from build123d import *

# Parameters (mm, degrees)
F0_W           = 220
F0_H           = 100
F0_R           = 0.625
F0_W_2         = 50
F0_H_2         = 80
F0_R_2         = 0.6265
F1_DEPTH       = 6.6
F2_SIZE2       = 2
F2_SIZE        = 2
F3_D           = 6.8
F4_D           = 6.6
F4_CBORE_D     = 11.25
F4_CBORE_DEPTH = 6
F5_R           = 10
F6_SIZE2       = 2
F6_SIZE        = 2


# Not quite as in the source:
# - a feature names something its author has since deleted; it is built from what else it names


with BuildPart() as f1:
    # F0 (on Top) → F1 (new body)
    with BuildSketch(Plane.XY):
        with Locations((-110, -50)):
            Rectangle(F0_W, F0_H)
        with Locations((-157.5, -70)):
            Circle(F0_R, mode=Mode.SUBTRACT)
        with Locations((-182.5, -30)):
            Circle(F0_R, mode=Mode.SUBTRACT)
        with Locations((-110, -50)):
            Rectangle(F0_W_2, F0_H_2, mode=Mode.SUBTRACT)
        with Locations((-37.5, -42.5)):
            Circle(F0_R_2, mode=Mode.SUBTRACT)
        with Locations((-62.5, -17.5)):
            Circle(F0_R, mode=Mode.SUBTRACT)
    extrude(amount=-F1_DEPTH)

    # F2
    f2_edges = [f1.edges().sort_by_distance(p)[0] for p in [
        (-110, -100, 0),
        (0, -50, 0),
        (-110, 0, 0),
        (-220, -50, 0),
    ]]
    chamfer(f2_edges, length=F2_SIZE, length2=F2_SIZE2)

    # F3 (through all)
    with Locations(Plane.XY):
        with Locations((-182.5, -30), (-157.5, -70), (-37.5, -42.5), (-62.5, -17.5)):
            Hole(F3_D / 2)

    # F4 (through all)
    with Locations(Plane.XY):
        with Locations((-210, -10), (-210, -90), (-10, -90), (-10, -10)):
            CounterBoreHole(F4_D / 2, F4_CBORE_D / 2, F4_CBORE_DEPTH)

    # F5
    f5_edges = [f1.edges().sort_by_distance(p)[0] for p in [
        (-135, -10, -3.3),
        (-85, -10, -3.3),
        (-135, -90, -3.3),
        (-85, -90, -3.3),
    ]]
    fillet(f5_edges, radius=F5_R)

    # F6
    f6_edges = [f1.edges().sort_by_distance(p)[0] for p in [
        (-135, -50, 0),
    ]]
    chamfer(f6_edges, length=F6_SIZE, length2=F6_SIZE2)


solid = f1.part
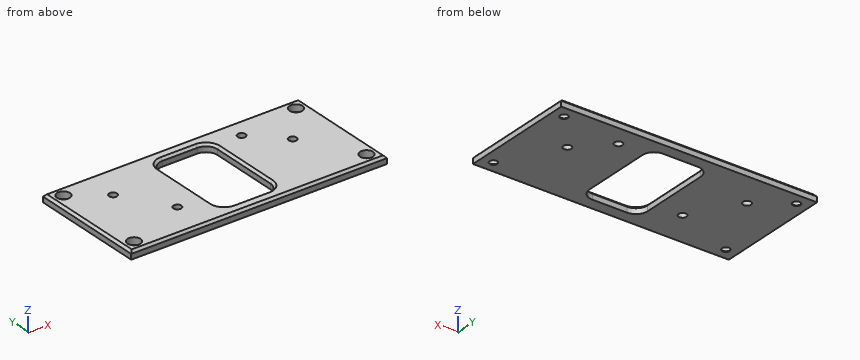
Design review of the part built by this model. Coordinates are the model's own, in mm. Give positions to 0.01 mm unless a question says otherwise; leave off trailing zeros. Loops run counter-clockwise (first coordinate to the right, second up) from the corner with the lowest first, then second, coordinate; pieces in that order, holes last. Notation, with made-up numbers: M 32,-18.75 L 83,-18.75 A20 cw 83,-8.75 Z; hole C 58.25,69.5 d11. An arc over 180 degrees is marked long. One line per question, with ' | ' between items. Start each with the question number.
1. To check wall thickness, follow L1, parallel to Y at x = -210, z = -6.1; L2, parallel to X at y = -38, z = -4; L3, parallel to X at y = -31.5, z = -4.75. State the ranges of each line that lie inside material, in increasing order.
2. Add section A-A (y = -42.5). Write out the cut boundary in (x, z).
3. Insertion check: P1, Ø3.5, axis at x = -9, y = -92.5, coming from the +Z side. The pin has a flat end and moves straight along its axis. Give the tip position at first contact, or say it passes through.
4. Add section D-D (z = -1). Give the number of separate pieces and of enclosed holes in the cut face, plus the area to 3 significant figures.
5. Add section C-C (x = -210). Write out the cut boundary in (y, z) (3 decimals).
6. Add section B-B (y = -23.5). Write out the cut boundary in (x, z), plus the area to 3 significant figures.
Worked out:
1) L1: y = -100 to -93.3, -86.7 to -13.3, -6.7 to 0 | L2: x = -220 to -135, -85 to 0 | L3: x = -220 to -185.55, -179.45 to -135, -85 to 0
2) outline: M -220,-6.6 L -135,-6.6 L -135,-2 L -137,0 L -218,0 L -220,-2 Z; M -85,-6.6 L -40.9,-6.6 L -40.9,0 L -83,0 L -85,-2 Z; M -34.1,-6.6 L 0,-6.6 L 0,-2 L -2,0 L -34.1,0 Z
3) P1: stops at z = -6
4) separate pieces: 1 | enclosed holes: 9 | area: 16,700 mm²
5) outline: M -100,-6.6 L -93.3,-6.6 L -93.3,-6 L -95.625,-6 L -95.625,0 L -98,0 L -100,-2 Z; M -86.7,-6.6 L -13.3,-6.6 L -13.3,-6 L -15.625,-6 L -15.625,0 L -84.375,0 L -84.375,-6 L -86.7,-6 Z; M -6.7,-6.6 L 0,-6.6 L 0,-2 L -2,0 L -4.375,0 L -4.375,-6 L -6.7,-6 Z
6) outline: M -220,-6.6 L -135,-6.6 L -135,-2 L -137,0 L -218,0 L -220,-2 Z; M -85,-6.6 L 0,-6.6 L 0,-2 L -2,0 L -83,0 L -85,-2 Z | area: 1,110 mm²
